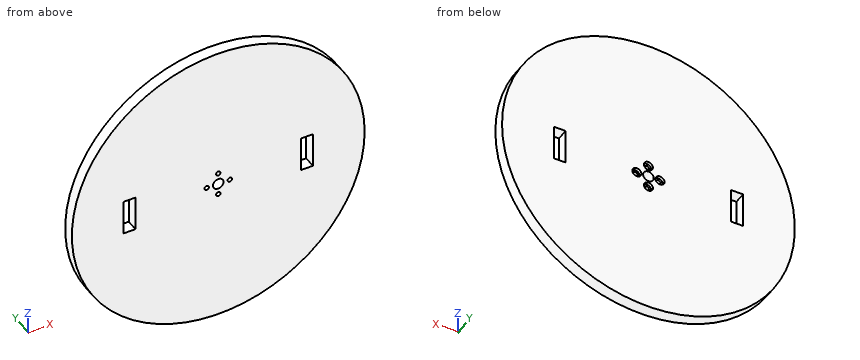
```python
from build123d import *

# Parameters (mm, degrees)
SKETCH1_R           = 123.75
BOSS_EXTRUDE1_DEPTH = 10
SKETCH2_R           = 1.905
CUT_EXTRUDE2_DEPTH  = 11
CIRPATTERN1_COUNT   = 4
SKETCH3_R           = 4.5
CUT_EXTRUDE3_DEPTH  = 11
SKETCH4_R           = 3.81
CUT_EXTRUDE4_DEPTH  = 2.54
CIRPATTERN2_COUNT   = 4
SKETCH5_W           = 10
SKETCH5_H           = 30
CUT_EXTRUDE5_DEPTH  = 11


with BuildPart() as part:
    # Sketch1 → Boss-Extrude1 (new body)
    with BuildSketch(Plane(origin=(0, 0, 0), x_dir=(1, 0, 0), z_dir=(0, 1, 0))):
        Circle(SKETCH1_R)
    extrude(amount=BOSS_EXTRUDE1_DEPTH)

    # Sketch2 → Cut-Extrude2 (cut, through all)
    with BuildSketch(Plane(origin=(0, 10, 0), x_dir=(1, 0, 0), z_dir=(0, 1, 0))):
        with Locations((0, 9.779)):
            Circle(SKETCH2_R)
    cut_extrude2 = extrude(amount=-CUT_EXTRUDE2_DEPTH, mode=Mode.SUBTRACT)

    # CirPattern1: Cut-Extrude2 ×4 about axis
    cirpattern1_axis = Axis((0, 0, 0), (0, 1, 0))
    for i in range(1, CIRPATTERN1_COUNT):
        add(cut_extrude2.rotate(cirpattern1_axis, i * 360 / CIRPATTERN1_COUNT), mode=Mode.SUBTRACT)

    # Sketch3 → Cut-Extrude3 (cut, through all)
    with BuildSketch(Plane(origin=(0, 10, 0), x_dir=(1, 0, 0), z_dir=(0, 1, 0))):
        Circle(SKETCH3_R)
    extrude(amount=-CUT_EXTRUDE3_DEPTH, mode=Mode.SUBTRACT)

    # Sketch4 → Cut-Extrude4 (cut)
    with BuildSketch(Plane(origin=(0, 10, 0), x_dir=(1, 0, 0), z_dir=(0, 1, 0))):
        with Locations((0, 9.779)):
            Circle(SKETCH4_R)
    cut_extrude4 = extrude(amount=-CUT_EXTRUDE4_DEPTH, mode=Mode.SUBTRACT)

    # CirPattern2: Cut-Extrude4 ×4 about axis
    cirpattern2_axis = Axis((0, 0, 0), (0, 1, 0))
    for i in range(1, CIRPATTERN2_COUNT):
        add(cut_extrude4.rotate(cirpattern2_axis, i * 360 / CIRPATTERN2_COUNT), mode=Mode.SUBTRACT)

    # Sketch5 → Cut-Extrude5 (cut, through all)
    with BuildSketch(Plane(origin=(0, 10, 0), x_dir=(1, 0, 0), z_dir=(0, 1, 0))):
        with Locations((75, 0)):
            Rectangle(SKETCH5_W, SKETCH5_H)
        with Locations((-75, 0)):
            Rectangle(SKETCH5_W, SKETCH5_H)
    extrude(amount=-CUT_EXTRUDE5_DEPTH, mode=Mode.SUBTRACT)


solid = part.part
```
Part model, mm, in its own coordinate system. Round coordinates to 2 decimals unless told otherwise and drop trailing zeros. Loops run counter-clockwise (first coordinate to the right, second up) from the corner with the lowest first, then second, coordinate; pieces in that order, holes last.
1. Slice it at C-C (x = -52.5). Give the cut face in (y, z), and give its area (3 significant figures).
Solutions:
outline: (0, -112.06) - (10, -112.06) - (10, 112.06) - (0, 112.06) - close
area: 2,240 mm2
2. Flat gauge pins, fed straight in: pin 1 (4.5 mm diameter, centred on x = -9.779, z = 0, fed in from +Y); pin 2 (8 mm diameter, centred on x = 0, z = 0, fed in from -Y); pin 3 (4 mm diameter, centred on x = 33.5, y = 6.5, fed in from -Z); pin 4 (5 mm diameter, centred on x = -74.5, y = 6, fed in from +Z). Where does each tip first touch, or does it go through?
Solutions:
pin 1: stops at y = 7.46
pin 2: passes through
pin 3: stops at z = -119.67
pin 4: stops at z = 100.65
3. Drill centre lines: line 1 along X through (y, z) = (5, 0); line 2 along Z through (x, y) = (0, 7); line 3 along X through (y, z) = (8.5, 0). Where is each one in solid material? Low to high.
Solutions:
line 1: x = -123.75 to -80, -70 to -11.68, -7.87 to -4.5, 4.5 to 7.87, 11.68 to 70, 80 to 123.75
line 2: z = -123.75 to -11.68, -7.87 to -4.5, 4.5 to 7.87, 11.68 to 123.75
line 3: x = -123.75 to -80, -70 to -13.59, -5.97 to -4.5, 4.5 to 5.97, 13.59 to 70, 80 to 123.75
4. Slice it at B-B (z = -66). Give the cut face in (x, y).
Solutions:
outline: (-104.68, 0) - (104.68, 0) - (104.68, 10) - (-104.68, 10) - close
5. Slice it at A-A (y = 5.5). Give the cut face in (x, z) (3 decimals).
Solutions:
outline: circle Ø247.5 at (0, 0); hole (-80, -15) - (-70, -15) - (-70, 15) - (-80, 15) - close; hole circle Ø3.81 at (-9.779, 0); hole circle Ø9 at (0, 0); hole circle Ø3.81 at (0, -9.779); hole circle Ø3.81 at (0, 9.779); hole circle Ø3.81 at (9.779, 0); hole (70, -15) - (80, -15) - (80, 15) - (70, 15) - close
